Work out the finished part from the listing and answer in its coordinate system (mm). A direction names the side the tool comes from. Round coordinates to 2 decimals unless told otherwise and drop trailing zeros. Loops run counter-clockwise (first coordinate to the right, second up) from the corner with the lowest first, then second, coordinate; pieces in that order, holes last. Notation, with made-up numbers: (76, 34.25) -> (107, 34.25) arc R25 cw to (107, 56.25) -> close; hole circle Ø4 at (-13.5, -13). An arc over 180 degrees is marked (long way). Use CSV: the item, a comma, the result in double quotes. Start each with the question number.
from build123d import *

# Parameters (mm, degrees)
SKETCH_R              = 150
PAD_DEPTH             = 6
SKETCH001_R           = 6
POCKET_DEPTH          = 854.613986
SKETCH002_W           = 30
SKETCH002_H           = 46
POCKET001_DEPTH       = 854.613986
POLARPATTERN_COUNT    = 12
POLARPATTERN001_COUNT = 2


with BuildPart() as part:
    # Sketch → Pad (new body)
    with BuildSketch(Plane.XY):
        Circle(SKETCH_R)
    extrude(amount=PAD_DEPTH)

    # Sketch001 (on Face3 of Pad) → Pocket (cut, through all)
    with BuildSketch(Plane.XY.offset(6)):
        with Locations((0, 50)):
            Circle(SKETCH001_R)
    pocket = extrude(amount=-POCKET_DEPTH, mode=Mode.SUBTRACT)

    # Sketch002 (on Face3 of Pocket) → Pocket001 (cut, through all)
    with BuildSketch(Plane.XY.offset(6)):
        with Locations((0, 127)):
            Rectangle(SKETCH002_W, SKETCH002_H)
    pocket001 = extrude(amount=-POCKET001_DEPTH, mode=Mode.SUBTRACT)

    # PolarPattern: Pocket001 ×12 about axis
    polarpattern_axis = Axis((0, 0, 6), (0, 0, 1))
    for i in range(1, POLARPATTERN_COUNT):
        add(pocket001.rotate(polarpattern_axis, i * 360 / POLARPATTERN_COUNT), mode=Mode.SUBTRACT)

    # PolarPattern001: Pocket ×2 about axis
    polarpattern001_axis = Axis((0, 0, 6), (0, 0, 1))
    for i in range(1, POLARPATTERN001_COUNT):
        add(pocket.rotate(polarpattern001_axis, i * 360 / POLARPATTERN001_COUNT), mode=Mode.SUBTRACT)


solid = part.part
Q1. Which of the six approach directions +Z, -Z, +X, -X, +Y, -Y give full straight-line access (tool end or side, diameter ignored) to faces 4 (the flat face through (-76.144, 101.885, 3.042)), 5 (the flat face through (51.82, 90.17, 3.04)), 6 (the flat face through (76.144, -101.885, 3.042)), 7 (the cylindrical face through (-105.826, 106.306, 2.958)), 8 (the flat face through (-101.885, 76.144, 3.042))?
Q2. Section B-B, the plane y = -50 is taken. Write down the section's boundary in (x, z), and give its area (3 significant figures).
Q3. For a pull along X with two mould halves and no side action, classify faces 1 (the flat face through (101.885, 76.144, 3.042)), 2 (the flat face through (-89.962, -52.182, 3.042)), 3 (the cylindrical face through (-39.15, -144.8, 2.96)) as pulls with the +X half, pulls with the -X half, needs draft (parallel to the pull), parting line crosses it, or undercut.
Q4. Section C-C, the plane z = 3.75 is taken. Give the number of separate pieces and of enclosed holes in the cut face, and give its area (3 significant figures).
Q5. Straight lines are drawn through the part: line 1 (Y direction, x = 0, z = 4.5); line 2 (X direction, y = -50, z = 4.6); line 3 (X direction, y = 54.5, z = 1.5). For each, find the intervals that lie inside material, in ascending order. Write a range as from..to.
Q6. Section D-D, the plane x = 111.5 is taken. Write down the section's boundary in (y, z), and give its area (3 significant figures).
Q7. Section A-A, the plane x = 0 is taken. Write down the section's boundary in (y, z).
Q8. Each of these flat-tipped pins is pushed along its axis until it touches: pin 1 (3 mm diameter, centred on y = 134, z = 4, fed in from -X); pin 2 (1.8 mm diameter, centred on y = -5, z = 3, fed in from -X); pin 3 (3 mm diameter, centred on y = -36.5, z = 3.5, fed in from +X). Where does it stop, or does it pass through?
Report:
1,face 4,"+Z, -Z, +Y"
1,face 5,"+Z, -Z"
1,face 6,"+Z, -Z, -Y"
1,face 7,"+Z, -Z, -X, +Y"
1,face 8,"+Z, -Z, -X"
2,outline,"(-141.42, 0) -> (-116.6, 0) -> (-116.6, 6) -> (-141.42, 6) -> close; (-91.22, 0) -> (-6, 0) -> (-6, 6) -> (-91.22, 6) -> close; (6, 0) -> (91.22, 0) -> (91.22, 6) -> (6, 6) -> close; (116.6, 0) -> (141.42, 0) -> (141.42, 6) -> (116.6, 6) -> close"
2,area,"1,320 mm²"
3,face 1,"pulls with the +X half"
3,face 2,"undercut"
3,face 3,"pulls with the -X half"
4,separate pieces,"1"
4,enclosed holes,"2"
4,area,"54,000 mm²"
5,line 1,"y = -104..-56, -44..44, 56..104"
5,line 2,"x = -141.42..-116.6, -91.22..-6, 6..91.22, 116.6..141.42"
5,line 3,"x = -139.75..-124.4, -88.62..-3.97, 3.97..88.62, 124.4..139.75"
6,outline,"(-100.34, 0) -> (-81.7, 0) -> (-81.7, 6) -> (-100.34, 6) -> close; (-47.05, 0) -> (-15, 0) -> (-15, 6) -> (-47.05, 6) -> close; (15, 0) -> (47.05, 0) -> (47.05, 6) -> (15, 6) -> close; (81.7, 0) -> (100.34, 0) -> (100.34, 6) -> (81.7, 6) -> close"
6,area,"608 mm²"
7,outline,"(-104, 0) -> (-56, 0) -> (-56, 6) -> (-104, 6) -> close; (-44, 0) -> (44, 0) -> (44, 6) -> (-44, 6) -> close; (56, 0) -> (104, 0) -> (104, 6) -> (56, 6) -> close"
8,pin 1,"stops at x = -60.91"
8,pin 2,"stops at x = -104"
8,pin 3,"stops at x = 145.86"
